```python
from build123d import *

# Parameters (mm, degrees)
F0_R      = 2
F1_DEPTH  = 1.5
F2_R      = 2.4
F2_R_2    = 2
F3_DEPTH  = 1.25
F4_SIZE   = 0.8
F6_DEPTH  = 23.5
F7_R      = 3.35
F8_DEPTH  = 1.5
F9_R      = 1.5
F10_DEPTH = 3


with BuildPart() as f1:
    # F0 (on Top) → F1 (new body)
    with BuildSketch(Plane.XY):
        Circle(F0_R)
    extrude(amount=F1_DEPTH)

    # F2 (on face) → F3 (join)
    with BuildSketch(Plane.XY.offset(1.5)):
        Circle(F2_R)
        Circle(F2_R_2, mode=Mode.SUBTRACT)
        Circle(F2_R_2)
    extrude(amount=F3_DEPTH)

    # F4
    f4_edges = [f1.edges().sort_by_distance(p)[0] for p in [
        (-2.4, 0, 2.75),
    ]]
    chamfer(f4_edges, length=F4_SIZE)

    # F5 (on face) → F6 (join)
    with BuildSketch(Plane(origin=(0, 0, 0), x_dir=(1, 0, 0), z_dir=(0, 0, -1))):
        with BuildLine():
            ThreePointArc((0.75, -1.85405), (0, -2), (-0.75, -1.85405))
            Line((-0.75, -1.85405), (-0.75, -2.5))
            Line((-0.75, -2.5), (0, -2.5))
            Line((0, -2.5), (0.75, -2.5))
            Line((0.75, -2.5), (0.75, -1.85405))
        make_face()
        with BuildLine():
            Line((-2.5, 0.75), (-2.5, 0))
            Line((-2.5, 0), (-2.5, -0.75))
            Line((-2.5, -0.75), (-1.85405, -0.75))
            ThreePointArc((-1.85405, -0.75), (-2, 0), (-1.85405, 0.75))
            Line((-1.85405, 0.75), (-2.5, 0.75))
        make_face()
        with BuildLine():
            Line((-0.75, 2.5), (-0.75, 1.85405))
            ThreePointArc((-0.75, 1.85405), (0, 2), (0.75, 1.85405))
            Line((0.75, 1.85405), (0.75, 2.5))
            Line((0.75, 2.5), (0, 2.5))
            Line((0, 2.5), (-0.75, 2.5))
        make_face()
        with BuildLine():
            ThreePointArc((2, 0), (1.963173, -0.382035), (1.85405, -0.75))
            Line((1.85405, -0.75), (2.5, -0.75))
            Line((2.5, -0.75), (2.5, 0))
            Line((2.5, 0), (2.5, 0.75))
            Line((2.5, 0.75), (1.85405, 0.75))
            ThreePointArc((1.85405, 0.75), (1.963173, 0.382035), (2, 0))
        make_face()
        with BuildLine():
            ThreePointArc((-1.85405, 0.75), (-2, 0), (-1.85405, -0.75))
            Line((-1.85405, -0.75), (-0.75, -0.75))
            Line((-0.75, -0.75), (-0.75, -1.85405))
            ThreePointArc((-0.75, -1.85405), (0, -2), (0.75, -1.85405))
            Line((0.75, -1.85405), (0.75, -0.75))
            Line((0.75, -0.75), (1.85405, -0.75))
            ThreePointArc((1.85405, -0.75), (1.963173, -0.382035), (2, 0))
            ThreePointArc((2, 0), (1.963173, 0.382035), (1.85405, 0.75))
            Line((1.85405, 0.75), (0.75, 0.75))
            Line((0.75, 0.75), (0.75, 1.85405))
            ThreePointArc((0.75, 1.85405), (0, 2), (-0.75, 1.85405))
            Line((-0.75, 1.85405), (-0.75, 0.75))
            Line((-0.75, 0.75), (-1.85405, 0.75))
        make_face()
    extrude(amount=F6_DEPTH)

    # F7 (on face) → F8 (join)
    with BuildSketch(Plane(origin=(0, 0, -23.5), x_dir=(1, 0, 0), z_dir=(0, 0, -1))):
        Circle(F7_R)
        Polygon((0.75, -2.5), (-0.75, -2.5), (-0.75, -0.75), (-2.5, -0.75), (-2.5, 0.75), (-0.75, 0.75), (-0.75, 2.5), (0.75, 2.5), (0.75, 0.75), (2.5, 0.75), (2.5, -0.75), (0.75, -0.75), align=None, mode=Mode.SUBTRACT)
        Polygon((-0.75, -0.75), (-0.75, -2.5), (0.75, -2.5), (0.75, -0.75), (2.5, -0.75), (2.5, 0.75), (0.75, 0.75), (0.75, 2.5), (-0.75, 2.5), (-0.75, 0.75), (-2.5, 0.75), (-2.5, -0.75), align=None)
    extrude(amount=F8_DEPTH)

    # F9 (on face) → F10 (join)
    with BuildSketch(Plane(origin=(0, 0, -25), x_dir=(1, 0, 0), z_dir=(0, 0, -1))):
        Circle(F9_R)
    extrude(amount=F10_DEPTH)


solid = f1.part
```
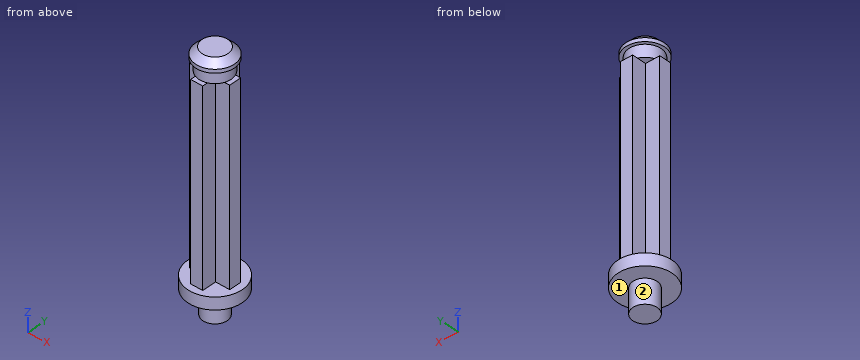
Model file for the job. Use its own axes, mm. Face numbers are marked on the shaded views. Give positions to 0.01 mm unless a question says otherwise; leave off trailing zeros. Write each loop counter-clockwise with the first axis right and the second up, starting at its lowest first coordinate (ties: lowest second). Pieces come first, ordered by that corner, then holes. Notation, with made-up numbers: M 58,-37 L 109,-37 A16 ccw 109,-13 Z; hole C 20,-35 d11. An arc over 180 degrees is marked long. Use a Markdown table: item, result.
1) Pull direction Y, two halves, no side cores. Call the marked faces 1 and 2: +Y half, -Y half, draft (parallel to the pull), parting line (faces both ways), or undercut.
Responses:
| item | result |
|---|---|
| face 1 | draft |
| face 2 | parting line |
2) Drill centre lines: line 1 (X direction, y = 0, z = -7.5); line 2 (Z direction, x = -3, y = -1.25); line 3 (X direction, y = -1.25, z = -16). Where is each one in solid material? Low to high. Write a range as from..to.
Responses:
| item | result |
|---|---|
| line 1 | x = -2.5..2.5 |
| line 2 | z = -25..-23.5 |
| line 3 | x = -0.75..0.75 |
3) Cut at D-D (x = 3). List the corners of the cut face in (y, z).
Responses:
| item | result |
|---|---|
| outline | M -1.49,-25 L 1.49,-25 L 1.49,-23.5 L -1.49,-23.5 Z |
4) Pin check, flat tips, straight feed: pin 1 (0.9 mm diameter, centred on x = 1.5, z = -8.5, fed in from +Y); pin 2 (3 mm diameter, centred on y = 1.5, z = -18.5, fed in from +X); pin 3 (2 mm diameter, centred on x = -2.5, y = 1, fed in from +Z). Stop position of each tip, or through.
Responses:
| item | result |
|---|---|
| pin 1 | stops at y = 0.75 |
| pin 2 | stops at x = 2.5 |
| pin 3 | stops at z = 2.66 |
5) Cut at A-A (x = 0). List the corners of the cut face in (y, z).
Responses:
| item | result |
|---|---|
| outline | M -3.35,-25 L -1.5,-25 L -1.5,-28 L 1.5,-28 L 1.5,-25 L 3.35,-25 L 3.35,-23.5 L 2.5,-23.5 L 2.5,0 L 2,0 L 2,1.5 L 2.4,1.5 L 2.4,1.95 L 1.6,2.75 L -1.6,2.75 L -2.4,1.95 L -2.4,1.5 L -2,1.5 L -2,0 L -2.5,0 L -2.5,-23.5 L -3.35,-23.5 Z |
6) Cut at B-B (z = -8). List the corners of the cut face in (x, y), and give its area (4 significant figures).
Responses:
| item | result |
|---|---|
| outline | M -2.5,-0.75 L -0.75,-0.75 L -0.75,-2.5 L 0.75,-2.5 L 0.75,-0.75 L 2.5,-0.75 L 2.5,0.75 L 0.75,0.75 L 0.75,2.5 L -0.75,2.5 L -0.75,0.75 L -2.5,0.75 Z |
| area | 12.75 mm2 |
